The model under review builds one solid part; all positions refer to its coordinate system, in mm. A direction names the side the tool comes from. Give positions to 0.01 mm unless a question says otherwise; leave off trailing zeros. Loops run counter-clockwise (first coordinate to the right, second up) from the corner with the lowest first, then second, coordinate; pieces in that order, holes last. Notation, with made-up numbers: M 65,24 L 102,24 A17 ccw 102,42 Z; hole C 89.5,74.5 d7. An arc over 180 degrees is marked long. Put each result on its own line as item: value. Start each with the question number.
from build123d import *

# Parameters (mm, degrees)
SKETCH2_W                = 50.8
SKETCH2_H                = 25.4
SKETCH2_W_2              = 44.45
SKETCH2_H_2              = 19.05
EXTRUDE_THIN1_DEPTH      = 457.2
SKETCH25_W               = 50.8
SKETCH25_H               = 25.4
SKETCH25_W_2             = 44.45
SKETCH25_H_2             = 19.05
BOSS_EXTRUDE14_DEPTH     = 25.4
SKETCH29_W               = 50.8
SKETCH29_H               = 25.4
SKETCH29_W_2             = 44.45
SKETCH29_H_2             = 19.05
CUT_EXTRUDE10_DEPTH      = 203.2
SKETCH34_R               = 9.779
SKETCH34_R_2             = 2.15265
CUT_EXTRUDE15_DEPTH      = 25.4
SKETCH35_W               = 50.8
SKETCH35_H               = 25.4
CUT_EXTRUDE16_DEPTH      = 76.2
SKETCH31_R               = 2.15265
CUT_EXTRUDE12_DEPTH      = 1
CUT_EXTRUDE12_DEPTH_BACK = 26.4


with BuildPart() as part:
    # Sketch2 → Extrude-Thin1 (new body)
    with BuildSketch(Plane(origin=(0, 0, 0), x_dir=(1, 0, 0), z_dir=(0, 1, 0))):
        with Locations((10.213756614, 0.671957672)):
            Rectangle(SKETCH2_W, SKETCH2_H)
        with Locations((10.213756614, 0.671957672)):
            Rectangle(SKETCH2_W_2, SKETCH2_H_2, mode=Mode.SUBTRACT)
    extrude(amount=EXTRUDE_THIN1_DEPTH)

    # Sketch25 → Boss-Extrude14 (add)
    with BuildSketch(Plane.XZ):
        with Locations((10.213756614, -0.671957672)):
            Rectangle(SKETCH25_W, SKETCH25_H)
        with Locations((10.213756614, -0.671957672)):
            Rectangle(SKETCH25_W_2, SKETCH25_H_2, mode=Mode.SUBTRACT)
    extrude(amount=BOSS_EXTRUDE14_DEPTH)

    # Sketch29 → Cut-Extrude10 (cut)
    with BuildSketch(Plane(origin=(0, 457.2, 0), x_dir=(1, 0, 0), z_dir=(0, 1, 0))):
        with Locations((10.213756614, 0.671957672)):
            Rectangle(SKETCH29_W, SKETCH29_H)
        with Locations((10.213756614, 0.671957672)):
            Rectangle(SKETCH29_W_2, SKETCH29_H_2, mode=Mode.SUBTRACT)
    extrude(amount=-CUT_EXTRUDE10_DEPTH, mode=Mode.SUBTRACT)

    # Sketch34 → Cut-Extrude15 (cut)
    with BuildSketch(Plane.XY.offset(12.028042328)):
        with Locations((10.213756614, 0)):
            Circle(SKETCH34_R)
        with Locations((29.263756614, 0)):
            Circle(SKETCH34_R_2)
        with Locations((23.684140795, 13.470384182)):
            Circle(SKETCH34_R_2)
        with Locations((10.213756614, 19.05)):
            Circle(SKETCH34_R_2)
        with Locations((-3.256627568, 13.470384182)):
            Circle(SKETCH34_R_2)
        with Locations((-8.836243386, 0)):
            Circle(SKETCH34_R_2)
        with Locations((-3.256627568, -13.470384182)):
            Circle(SKETCH34_R_2)
        with Locations((10.213756614, -19.05)):
            Circle(SKETCH34_R_2)
        with Locations((23.684140795, -13.470384182)):
            Circle(SKETCH34_R_2)
    extrude(amount=-CUT_EXTRUDE15_DEPTH, mode=Mode.SUBTRACT)

    # Sketch35 → Cut-Extrude16 (cut)
    with BuildSketch(Plane(origin=(0, 254, 0), x_dir=(1, 0, 0), z_dir=(0, 1, 0))):
        with Locations((10.213756614, 0.671957672)):
            Rectangle(SKETCH35_W, SKETCH35_H)
    extrude(amount=-CUT_EXTRUDE16_DEPTH, mode=Mode.SUBTRACT)

    # Sketch31 → Cut-Extrude12 (cut, two sides)
    with BuildSketch(Plane(origin=(0, 0, -13.371957672), x_dir=(-1, 0, 0), z_dir=(0, 0, -1))) as cut_extrude12_sk:
        with Locations((-19.738756614, 146.05)):
            Circle(SKETCH31_R)
        with Locations((-0.688756614, 146.05)):
            Circle(SKETCH31_R)
        with Locations((-19.738756614, 171.45)):
            Circle(SKETCH31_R)
        with Locations((-0.688756614, 171.45)):
            Circle(SKETCH31_R)
    extrude(amount=CUT_EXTRUDE12_DEPTH, mode=Mode.SUBTRACT)
    extrude(cut_extrude12_sk.sketch, amount=-CUT_EXTRUDE12_DEPTH_BACK, mode=Mode.SUBTRACT)


solid = part.part
(1) Draft analysis for pull direction Y (two halves, no side actions). For faces 3 (the cylindrical face through (27.113, 0.095, 10.463)), 4 (the flat face through (10, 78, 8.853)), state which applies: +Y half, -Y half, draft (parallel to the pull), parting line (faces both ways), or undercut.
(2) We need section A-A, the plane z = -5.25. Write out the cut boundary in (x, y), plus the area to 3 significant figures.
(3) For faces 1 (the cylindrical face through (21.976, -14.78, 10.463)), 2 (the flat face through (32.439, 78, -1)), list the 3-axis set-ups (+Z, -Z, +X, -X, +Y, -Y) from which the entire face can be reached by the end or side of a thin tool; tool diameter is ignored.
(4) We need section B-B, the plane y = 19.05. Write out the cut boundary in (x, z), plus the area to 3 significant figures.
(5) To check wall thickness, follow L1, parallel to Z at x = 9, y = 13; L2, parallel to X at y = 141.5, z = -3. State the ranges of each line that lie inside material, in increasing order. Write a range as [from, to].
(6) We need section D-D, the plane x = 29. Write out the cut boundary in (y, z), plus the area to 3 significant figures.
(7) We need section C-C, the plane y = 171.45. Write out the cut boundary in (x, z).
Check sheet entries:
1. face 3: undercut
1. face 4: draft
2. outline: M -15.19,-25.4 L -12.01,-25.4 L -12.01,177.8 L -15.19,177.8 Z; M 32.44,-25.4 L 35.61,-25.4 L 35.61,177.8 L 32.44,177.8 Z
2. area: 1,290 mm²
3. face 1: +Z, -Z
3. face 2: +Y, -Y
4. outline: M -15.19,-13.37 L 8.06,-13.37 L 8.06,-10.2 L -12.01,-10.2 L -12.01,8.85 L 8.06,8.85 L 8.06,12.03 L -15.19,12.03 Z; M 12.37,-13.37 L 35.61,-13.37 L 35.61,12.03 L 12.37,12.03 L 12.37,8.85 L 32.44,8.85 L 32.44,-10.2 L 12.37,-10.2 Z
4. area: 416 mm²
5. L1: z = [-13.37, -10.2], [8.85, 12.03]
5. L2: x = [-15.19, -12.01], [32.44, 35.61]
6. outline: M -25.4,-13.37 L -2.14,-13.37 L -2.14,-10.2 L -25.4,-10.2 Z; M -25.4,8.85 L -2.14,8.85 L -2.14,12.03 L -25.4,12.03 Z; M 2.14,-13.37 L 177.8,-13.37 L 177.8,-10.2 L 2.14,-10.2 Z; M 2.14,8.85 L 177.8,8.85 L 177.8,12.03 L 2.14,12.03 Z
6. area: 1,260 mm²
7. outline: M -15.19,-13.37 L -1.46,-13.37 L -1.46,-10.2 L -12.01,-10.2 L -12.01,8.85 L -1.46,8.85 L -1.46,12.03 L -15.19,12.03 Z; M 2.84,-13.37 L 17.59,-13.37 L 17.59,-10.2 L 2.84,-10.2 Z; M 2.84,8.85 L 17.59,8.85 L 17.59,12.03 L 2.84,12.03 Z; M 21.89,-13.37 L 35.61,-13.37 L 35.61,12.03 L 21.89,12.03 L 21.89,8.85 L 32.44,8.85 L 32.44,-10.2 L 21.89,-10.2 Z
